```python
from build123d import *

# Parameters (mm, degrees)
SKETCH1_R           = 73.4441
SKETCH1_R_2         = 67.0941
BOSS_EXTRUDE1_DEPTH = 9.525
CIRPATTERN1_COUNT   = 4


with BuildPart() as part:
    # Sketch1 → Boss-Extrude1 (new body)
    with BuildSketch(Plane(origin=(0, 0, 0), x_dir=(1, 0, 0), z_dir=(0, 1, 0))):
        Circle(SKETCH1_R)
        Circle(SKETCH1_R_2, mode=Mode.SUBTRACT)
    extrude(amount=BOSS_EXTRUDE1_DEPTH)

    # Sketch3 → Tap Drill for #4-40 Tap1 (revolve, cut)
    with BuildSketch(Plane(origin=(0, 4.7625, 73.4441), x_dir=(0, -1, 0), z_dir=(1, 0, 0))):
        Polygon((0, 0), (0, 5.441652758), (1.1303, 4.7625), (1.1303, 0), align=None)
    tap_drill_for_4_40_tap1 = revolve(axis=Axis((0, 4.7625, 79.7941), (0, 0, -1)), mode=Mode.SUBTRACT)

    # CirPattern1: Tap Drill for #4-40 Tap1 ×4 about axis
    cirpattern1_axis = Axis((0, 9.525, 0), (0, 1, 0))
    for i in range(1, CIRPATTERN1_COUNT):
        add(tap_drill_for_4_40_tap1.rotate(cirpattern1_axis, i * 360 / CIRPATTERN1_COUNT), mode=Mode.SUBTRACT)


solid = part.part
```
Could you check a few things on this model? Use its own coordinates, in mm. Round coordinates to 2 decimals unless told otherwise and drop trailing zeros. Loops run counter-clockwise (first coordinate to the right, second up) from the corner with the lowest first, then second, coordinate; pieces in that order, holes last. Notation, with made-up numbers: M -29.5,72 L -20.5,72 A15 cw -20.5,84 Z; hole C 78.25,-15 d3. An arc over 180 degrees is marked long. Answer as CSV lines item,"result".
1) If I drill on probe 1 along X at (y, z) = (6.25, 0); probe 2 along Y at (x, z) = (0, 70) (3 decimals); probe 3 along Z at (x, y) = (35, 5.25), over which ranges is the centre line in solid material (lowest first)?
From the geometry:
probe 1,"-73.44 to -67.09, 67.09 to 73.44"
probe 2,"0 to 3.632, 5.893 to 9.525"
probe 3,"-64.57 to -57.24, 57.24 to 64.57"
2) We'd pull the mould along X, two halves only. Please class faces 1 (the cylindrical face through (-15.921, 4.696, 71.698)), 2 (the cylindrical face through (-67.03, 4.7, -2.95)), 3 (the flat face through (32, 0, 60)): released by +X, released by -X, zero draft, split by the parting line, or undercut.
From the geometry:
face 1,"split by the parting line"
face 2,"undercut"
face 3,"zero draft"
3) Imagine slicing it at B-B on z = 31.5. List the corners of the cut face in (x, y) for me (3 decimals).
From the geometry:
outline,"M -66.346,0 L -59.24,0 L -59.24,9.525 L -66.346,9.525 Z; M 59.24,0 L 66.346,0 L 66.346,9.525 L 59.24,9.525 Z"
4) Imagine slicing it at A-A on x = 53.5. List the corners of the cut face in (y, z) for me (3 decimals).
From the geometry:
outline,"M 0,-50.317 L 9.525,-50.317 L 9.525,-40.489 L 0,-40.489 Z; M 0,40.489 L 9.525,40.489 L 9.525,50.317 L 0,50.317 Z"
5) For pin 1 Ø3 at (x, y) = (-44, 8) entering from +Z; pin 2 Ø3 at (x, y) = (54.5, 1.5) entering from -Z; pin 3 Ø5 at (y, z) = (7, 45.5) entering from +X, each with a flat end and sliding along its axis, tell me the tip position at first contact or that it passes through.
From the geometry:
pin 1,"z = 59.9"
pin 2,"z = -50.84"
pin 3,"x = 59.54"
